Model file for the job. Use its own axes, mm. Face numbers are marked on the shaded views. A direction names the side the tool comes from. Round coordinates to 2 decimals unless told otherwise and drop trailing zeros. Write each loop counter-clockwise with the first axis right and the second up, starting at its lowest first coordinate (ties: lowest second). Pieces come first, ordered by that corner, then holes. Notation, with made-up numbers: (63.25, 43.25) - (100.25, 43.25) arc R23 ccw to (100.25, 63.25) - close; hole circle Ø9 at (-19.75, 73). An arc over 180 degrees is marked (long way). Answer as a JSON object with one key per item and string values. Group by question number.
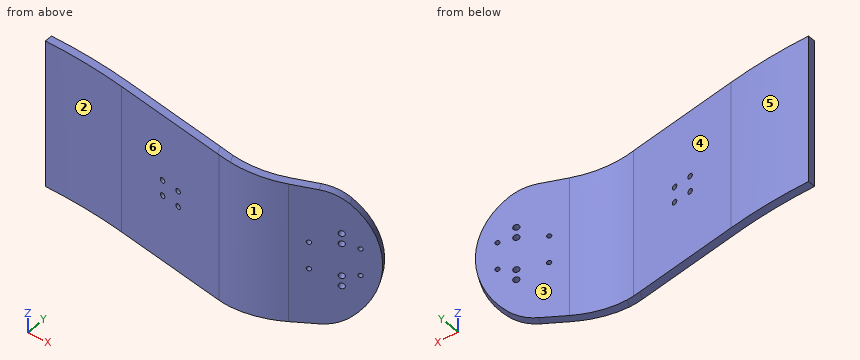
from build123d import *

# Parameters (mm, degrees)
EXTRUDE_THIN1_DEPTH  = 115
CUT_EXTRUDE1_DEPTH   = 620.892995583
FILLET1_R            = 250
SKETCH3_R            = 4
BINDING_HOLES_DEPTH  = 527.107084161
SKETCH4_R            = 4
CUT_EXTRUDE2_DEPTH   = 947.891927405
M6_CLEARANCE_HOLE1_D = 6.6
M8_CLEARANCE_HOLE1_D = 9
SKETCH9_W            = 500
SKETCH9_H            = 230
CUT_EXTRUDE3_DEPTH   = 520.361349661


with BuildPart() as part:
    # Sketch1 → Extrude-Thin1 (new, symmetric)
    with BuildSketch(Plane.XY):
        with BuildLine():
            Line((-500, 70), (-396.134492808, 17.077880761))
            ThreePointArc((-396.134492808, 17.077880761), (-349.336150967, 1.90144375), (-300.138569045, 1.984944587))
            Line((-300.138569045, 1.984944587), (-126.368172253, 29.91072477))
            ThreePointArc((-126.368172253, 29.91072477), (0, 40), (126.368172253, 29.91072477))
            Line((126.368172253, 29.91072477), (300.138569045, 1.984944587))
            ThreePointArc((300.138569045, 1.984944587), (349.336150967, 1.90144375), (396.134492808, 17.077880761))
            Line((396.134492808, 17.077880761), (500, 70))
            Line((500, 70), (494.552114003, 80.69207829))
            Line((494.552114003, 80.69207829), (390.686606812, 27.769959051))
            ThreePointArc((390.686606812, 27.769959051), (347.472349444, 13.755820321), (302.042599512, 13.832926187))
            Line((302.042599512, 13.832926187), (128.27220272, 41.75870637))
            ThreePointArc((128.27220272, 41.75870637), (0, 52), (-128.27220272, 41.75870637))
            Line((-128.27220272, 41.75870637), (-302.042599512, 13.832926187))
            ThreePointArc((-302.042599512, 13.832926187), (-347.472349444, 13.755820321), (-390.686606812, 27.769959051))
            Line((-390.686606812, 27.769959051), (-494.552114003, 80.69207829))
            Line((-494.552114003, 80.69207829), (-500, 70))
        make_face()
    extrude(amount=EXTRUDE_THIN1_DEPTH, both=True)

    # Sketch2 → Cut-Extrude1 (cut, symmetric)
    with BuildSketch(Plane(origin=(-69.290206127, -135.989686473, 0), x_dir=(-0.8910065241883677, 0.4539904997395473, 0), z_dir=(0.45399049973954725, 0.8910065241883676, 0))):
        with BuildLine():
            Line((-1243.954382633, 226.09395148), (275.40194382, 115))
            Line((275.40194382, 115), (398.488815391, 106))
            ThreePointArc((398.488815391, 106), (418.996120575, 101.069384919), (436.845066451, 89.8321405))
            ThreePointArc((436.845066451, 89.8321405), (477.282597076, 0), (436.845066451, -89.8321405))
            ThreePointArc((436.845066451, -89.8321405), (418.996120575, -101.069384919), (398.488815391, -106))
            Line((398.488815391, -106), (275.40194382, -115))
            Line((275.40194382, -115), (-1243.954382633, -226.09395148))
            Line((-1243.954382633, -226.09395148), (1802.870530478, -226.09395148))
            Line((1802.870530478, -226.09395148), (1802.870530478, 226.09395148))
            Line((1802.870530478, 226.09395148), (-1243.954382633, 226.09395148))
        make_face()
    cut_extrude1 = extrude(amount=CUT_EXTRUDE1_DEPTH, both=True, mode=Mode.SUBTRACT)

    # Mirror1: Cut-Extrude1 across plane
    add(cut_extrude1.mirror(Plane(origin=(0, 0, 0), x_dir=(0, 0, 1), z_dir=(1, 0, 0))), mode=Mode.SUBTRACT)

    # Fillet1
    # the kernel refuses this fillet: 250 mm, written as the material it takes off along each edge
    with BuildSketch(Plane(origin=(-319.014996724, -19.477278886, 115), x_dir=(-0.8886341933277065, 0.4527817367914195, -0.07292440796442752), z_dir=(0.45399049973954736, 0.8910065241883677, 0))) as fillet1_piece_1:
        with BuildLine():
            CenterArc((FILLET1_R * 0.0365108095299, -FILLET1_R), FILLET1_R, 90, 4.181973001)
            Line((-FILLET1_R * 0.0364135984345, -FILLET1_R * 0.00266252916927), (-FILLET1_R * 0.0378720865938, FILLET1_R * 0.0172842202473))
            Line((-FILLET1_R * 0.0378720865938, FILLET1_R * 0.0172842202473), (-FILLET1_R * 0.000730216190598, FILLET1_R * 0.02))
            Line((-FILLET1_R * 0.000730216190598, FILLET1_R * 0.02), (FILLET1_R * 0.0365108095299, FILLET1_R * 0.02))
            Line((FILLET1_R * 0.0365108095299, FILLET1_R * 0.02), (FILLET1_R * 0.0365108095299, 0))
        make_face()
    extrude(amount=60.204173091, mode=Mode.SUBTRACT)
    # the kernel refuses this fillet: 250 mm, written as the material it takes off along each edge
    with BuildSketch(Plane(origin=(319.014996724, -19.477278886, 115), x_dir=(-0.8910065241883677, -0.4539904997395473, 0), z_dir=(-0.45399049973954736, 0.8910065241883677, 0))) as fillet1_2_piece_1:
        with BuildLine():
            CenterArc((FILLET1_R * 0.0365108095299, -FILLET1_R), FILLET1_R, 90, 4.181973001)
            Line((-FILLET1_R * 0.0364135984345, -FILLET1_R * 0.00266252916927), (-FILLET1_R * 0.0378720865938, FILLET1_R * 0.0172842202473))
            Line((-FILLET1_R * 0.0378720865938, FILLET1_R * 0.0172842202473), (-FILLET1_R * 0.000730216190598, FILLET1_R * 0.02))
            Line((-FILLET1_R * 0.000730216190598, FILLET1_R * 0.02), (FILLET1_R * 0.0365108095299, FILLET1_R * 0.02))
            Line((FILLET1_R * 0.0365108095299, FILLET1_R * 0.02), (FILLET1_R * 0.0365108095299, 0))
        make_face()
    extrude(amount=60.204173091, mode=Mode.SUBTRACT)
    # the kernel refuses this fillet: 250 mm, written as the material it takes off along each edge
    with BuildSketch(Plane(origin=(-319.014996724, -19.477278886, -115), x_dir=(0.8910065241883677, -0.4539904997395473, 0), z_dir=(0.4539904997395473, 0.8910065241883677, 0))) as fillet1_3_piece_1:
        with BuildLine():
            CenterArc((FILLET1_R * 0.0365108095299, -FILLET1_R), FILLET1_R, 90, 4.181973001)
            Line((-FILLET1_R * 0.0364135984345, -FILLET1_R * 0.00266252916927), (-FILLET1_R * 0.0378720865938, FILLET1_R * 0.0172842202473))
            Line((-FILLET1_R * 0.0378720865938, FILLET1_R * 0.0172842202473), (-FILLET1_R * 0.000730216190598, FILLET1_R * 0.02))
            Line((-FILLET1_R * 0.000730216190598, FILLET1_R * 0.02), (FILLET1_R * 0.0365108095299, FILLET1_R * 0.02))
            Line((FILLET1_R * 0.0365108095299, FILLET1_R * 0.02), (FILLET1_R * 0.0365108095299, 0))
        make_face()
    extrude(amount=60.204173091, mode=Mode.SUBTRACT)
    # the kernel refuses this fillet: 250 mm, written as the material it takes off along each edge
    with BuildSketch(Plane(origin=(319.014996724, -19.477278886, -115), x_dir=(-0.8910065241883677, -0.4539904997395473, 0), z_dir=(-0.4539904997395473, 0.8910065241883677, 0))) as fillet1_4_piece_1:
        with BuildLine():
            CenterArc((FILLET1_R * 0.0365108095299, FILLET1_R), FILLET1_R, 265.818026999, 4.181973001)
            Line((-FILLET1_R * 0.0364135984345, FILLET1_R * 0.00266252916927), (-FILLET1_R * 0.0378720865938, -FILLET1_R * 0.0172842202473))
            Line((-FILLET1_R * 0.0378720865938, -FILLET1_R * 0.0172842202473), (-FILLET1_R * 0.000730216190598, -FILLET1_R * 0.02))
            Line((-FILLET1_R * 0.000730216190598, -FILLET1_R * 0.02), (FILLET1_R * 0.0365108095299, -FILLET1_R * 0.02))
            Line((FILLET1_R * 0.0365108095299, -FILLET1_R * 0.02), (FILLET1_R * 0.0365108095299, 0))
        make_face()
    extrude(amount=60.204173091, mode=Mode.SUBTRACT)

    # Sketch3 → Binding Holes (cut, through all)
    with BuildSketch(Plane(origin=(-9.771253847, 60.8024072, 0), x_dir=(-0.9873317999532861, -0.15866920558509276, 0), z_dir=(-0.15866920558509276, 0.9873317999532861, 0))):
        with Locations((222.02140403, 12)):
            Circle(SKETCH3_R)
        with Locations(Location((222.02140403, -12, 0), (0, 0, 180))):
            Circle(SKETCH3_R)
        with Locations((194.02140403, -12)):
            Circle(SKETCH3_R)
        with Locations(Location((194.02140403, 12, 0), (0, 0, 180))):
            Circle(SKETCH3_R)
    extrude(amount=-BINDING_HOLES_DEPTH, mode=Mode.SUBTRACT)

    # Sketch4 → Cut-Extrude2 (cut, through all)
    with BuildSketch(Plane(origin=(430.771006706, -6.854378838, -35.350500744), x_dir=(-0.9873317999532861, 0.15866920558509276, 0), z_dir=(0.15866920558509276, 0.9873317999532861, 0))):
        with Locations((232.380088234, 47.350500744)):
            Circle(SKETCH4_R)
        with Locations(Location((232.380088234, 23.350500744, 0), (0, 0, 180))):
            Circle(SKETCH4_R)
        with Locations((204.380088234, 23.350500744)):
            Circle(SKETCH4_R)
        with Locations(Location((204.380088234, 47.350500744, 0), (0, 0, 180))):
            Circle(SKETCH4_R)
    extrude(amount=-CUT_EXTRUDE2_DEPTH, mode=Mode.SUBTRACT)

    # M6 Clearance Hole1 (through all)
    with Locations(Plane(origin=(-49.331097603, -146.159360215, -63.345400331), x_dir=(-0.8910065241883677, 0.4539904997395473, 0), z_dir=(0.45399049973954725, 0.8910065241883676, 0))):
        with Locations((472.112244346, 84.345400331), (408.112244346, 84.345400331), (408.112244346, 42.345400331), (472.112244346, 42.345400331)):
            m6_clearance_hole1 = Hole(M6_CLEARANCE_HOLE1_D / 2)

    # M8 Clearance Hole1 (through all)
    with Locations(Plane(origin=(-70.616279149, -135.31401852, -54.210944478), x_dir=(-0.8910065241883677, 0.4539904997395473, 0), z_dir=(0.45399049973954725, 0.8910065241883676, 0))):
        with Locations((424.936326624, 95.560944478), (424.936326624, 79.560944478), (424.936326624, 12.860944478), (424.936326624, 28.860944478)):
            m8_clearance_hole1 = Hole(M8_CLEARANCE_HOLE1_D / 2)

    # Mirror2: M6 Clearance Hole1, M8 Clearance Hole1 across plane
    add(m6_clearance_hole1.mirror(Plane(origin=(0, 0, 0), x_dir=(0, 0, 1), z_dir=(1, 0, 0))), mode=Mode.SUBTRACT)
    add(m8_clearance_hole1.mirror(Plane(origin=(0, 0, 0), x_dir=(0, 0, 1), z_dir=(1, 0, 0))), mode=Mode.SUBTRACT)

    # Sketch9 → Cut-Extrude3 (cut, through all)
    with BuildSketch(Plane(origin=(0, 0, 0), x_dir=(1, 0, 0), z_dir=(0, 1, 0))):
        with Locations((-250, 0)):
            Rectangle(SKETCH9_W, SKETCH9_H)
    extrude(amount=CUT_EXTRUDE3_DEPTH, mode=Mode.SUBTRACT)


solid = part.part
(1) Pull direction X, two halves, no side cores. Call the marked faces 1, 2, 3 and 4: pulls with the +X half, pulls with the -X half, needs draft (parallel to the pull), parting line crosses it, or undercut.
(2) Drill centre lines: line 1 (Y direction, x = 326.5, z = -22); line 2 (Y direction, x = 409.5, z = 38); line 3 (X direction, y = 75, z = -45.5). Where is each one in solid material? Low to high. Write a range as from..to.
(3) 3-axis set-ups, long thin cutter, end or side, ignore diameter. For the marked faces 5 and 6: which of +Z, -Z, +X, -X, +Y, -Y reach the whole face in a straight line?
(4) Slice it at D-D (x = 51). Write the cut outline in (y, z), then the cut area to 3 significant figures.
(5) Slice it at A-A (z = -74.5). Write the cut outline in (x, y), then the cut area to 3 significant figures.
(6) Flat gauge pins, fed straight in: pin 1 (10 mm diameter, centred on x = 153, z = -2.5, fed in from +Y); pin 2 (5 mm diameter, centred on x = 335.5, z = -32, fed in from +Y); pin 3 (4 mm diameter, centred on x = 129.5, z = -74, fed in from -Y). Where does each tip first touch, or does it go through?
(7) Slice it at C-C (z = 96). Write the cut outline in (x, y).
(8) Slice it at B-B (x = 346). Write the cut outline in (y, z).
Answer:
{
 "1": {"face 1": "parting line crosses it", "face 2": "pulls with the -X half", "face 3": "undercut", "face 4": "undercut"},
 "2": {"line 1": "0.01..12.01", "line 2": "23.89..37.36", "line 3": "483.38..487.4"},
 "3": {"face 5": "+Z, -Z, +Y", "face 6": "+Z, -Z, -X, -Y"},
 "4": {"outline": "(38.37, -115) - (50.39, -115) - (50.39, 115) - (38.37, 115) - close", "area": "2,770 mm²"},
 "5": {"outline": "(0, 40) arc R796.43 cw to (126.37, 29.91) - (300.14, 1.98) arc R156.69 ccw to (396.13, 17.08) - (476.9, 58.23) - (471.45, 68.92) - (390.69, 27.77) arc R144.69 cw to (302.04, 13.83) - (128.27, 41.76) arc R808.43 ccw to (0, 52) - close", "area": "5,870 mm²"},
 "6": {"pin 1": "y = 38.59", "pin 2": "y = 12.59", "pin 3": "y = 29.09"},
 "7": {"outline": "(0, 40) arc R796.43 cw to (126.37, 29.91) - (300.14, 1.98) arc R156.69 ccw to (396.13, 17.08) - (456.68, 47.93) - (451.23, 58.62) - (390.69, 27.77) arc R144.69 cw to (302.04, 13.83) - (128.27, 41.76) arc R808.43 ccw to (0, 52) - close"},
 "8": {"outline": "(1.41, -112.55) - (13.53, -112.15) - (13.53, 112.15) - (1.41, 112.55) - close"}
}
